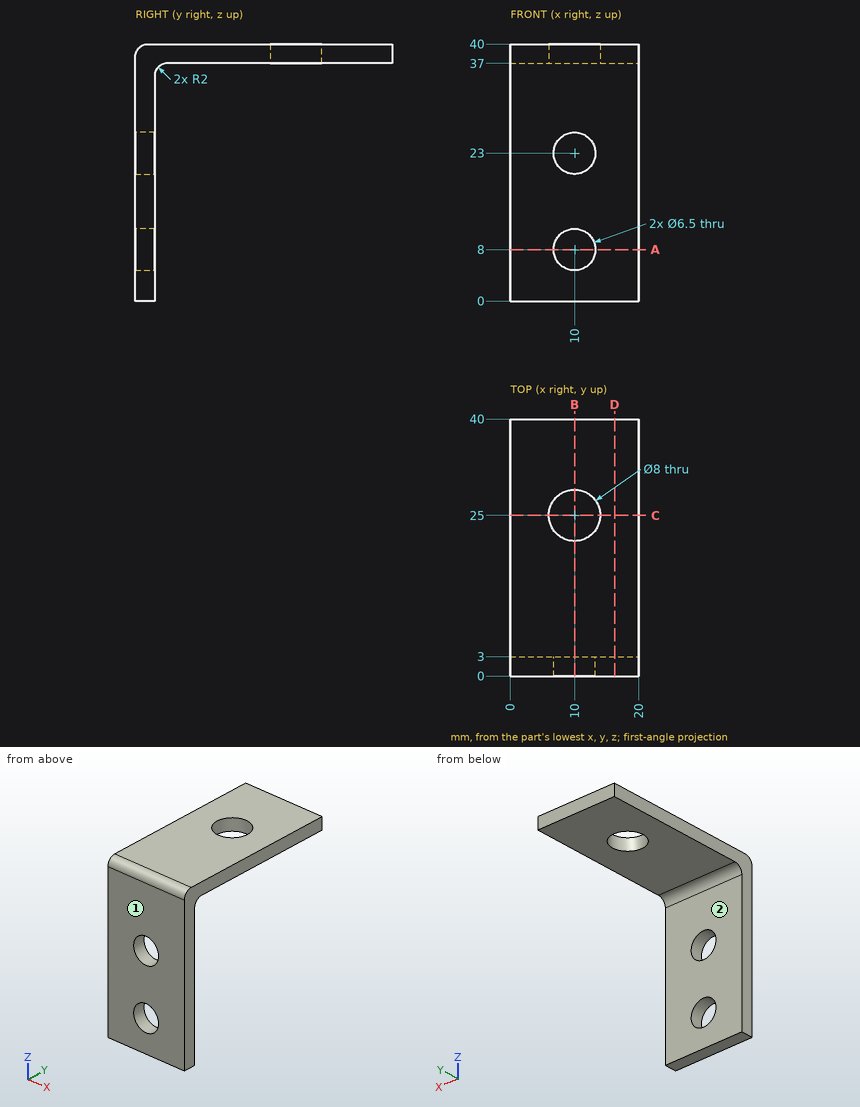
Part print with two shaded views. Sizes in mm from the minimum x, y, z corner. A direction names the side the tool comes from. Round coordinates to 2 decimals unless told otherwise and drop trailing zeros. Order: outer loops, then holes, each group sorted by start corner. A loop starts at its lowest first (then second) coordinate and runs counter-clockwise, first axis right, second up.
(1) Band-saw the part on B-B (x = 10). List the corners of the cut face in (y, z).
(2) Band-saw the part on D-D (x = 16.25). List the corners of the cut face in (y, z).
(3) 3-axis set-ups, long thin cutter, end or side, ignore diameter. For the marked faces 1 and 2: which of +Z, -Z, +X, -X, +Y, -Y reach the whole face in a straight line?
(4) Drill centre lines: line 1 (X direction, y = 1, z = 23); line 2 (X direction, y = 25, z = 37.8); line 3 (Y direction, x = 16.25, z = 29). Where is each one in solid material? Low to high.
(5) Band-saw the part on A-A (z = 8). List the corners of the cut face in (x, y), then the cut area to 3 significant figures.
(6) Band-saw the part on C-C (y = 25). List the corners of the cut face in (x, z), then the cut area to 3 significant figures.
(7) Pin check, flat tips, straight feed: pin 1 (3 mm diameter, centred on x = 7.5, z = 8, fed in from +Y); pin 2 (10 mm diameter, centred on x = 7.5, y = 16.5, fed in from -Z). Stop position of each tip, or through.
Verdict:
1. outline: (0, 0) - (3, 0) - (3, 4.75) - (0, 4.75) - close; (0, 11.25) - (3, 11.25) - (3, 19.75) - (0, 19.75) - close; (0, 26.25) - (3, 26.25) - (3, 35) arc R2 cw to (5, 37) - (21, 37) - (21, 40) - (2, 40) arc R2 ccw to (0, 38) - close; (29, 37) - (40, 37) - (40, 40) - (29, 40) - close
2. outline: (0, 0) - (3, 0) - (3, 35) arc R2 cw to (5, 37) - (40, 37) - (40, 40) - (2, 40) arc R2 ccw to (0, 38) - close
3. face 1: +Z, -Z, +X, -X, -Y
3. face 2: -Z, +X, -X, +Y
4. line 1: x = 0 to 6.75, 13.25 to 20
4. line 2: x = 0 to 6, 14 to 20
4. line 3: y = 0 to 3
5. outline: (0, 0) - (6.75, 0) - (6.75, 3) - (0, 3) - close; (13.25, 0) - (20, 0) - (20, 3) - (13.25, 3) - close
5. area: 40.5 mm2
6. outline: (0, 37) - (6, 37) - (6, 40) - (0, 40) - close; (14, 37) - (20, 37) - (20, 40) - (14, 40) - close
6. area: 36.0 mm2
7. pin 1: stops at y = 3
7. pin 2: stops at z = 37
